Study the drawing (mm; zero at the part's minimum x, y, z) and answer. Coordinates: 2 decimals unless noted, no trailing zeros. Order: outer loops, then holes, each group sorted by start corner. A loop starts at its lowest first (then second) coordinate and runs counter-clockwise, first axis right, second up.
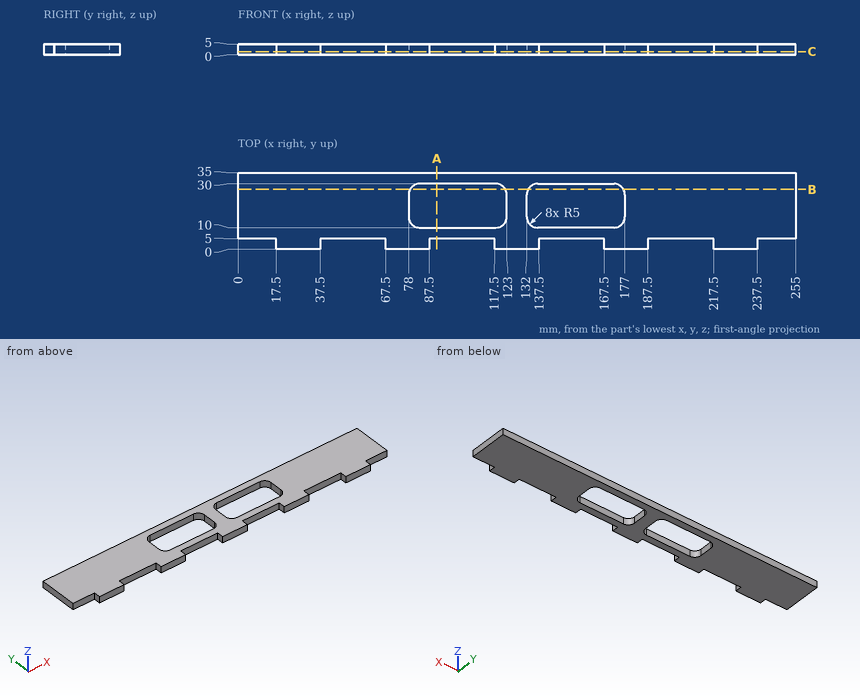
(1) Find the intervals of material crossed by probe 1 along X at (y, z) = (23.5, 2.3); probe 2 along X at (y, z) = (3.5, 4.1); probe 3 along Y at (x, z) = (97.5, 1.65), in increasing order.
(2) Given pin 1 Ø1.5 at (x, z) = (96, 1.5) entering from -Y; pin 2 Ø2.5 at (y, z) = (3.5, 3.5) entering from -X; pin 3 Ø2.5 at (y, z) = (3.5, 3) entering from +X, each flat-ended and moving along its own axis, determine where each tip first touches the part or whether it passes through.
(3) Find section B-B on y = 27.5. Determine the outline of the cut face in (x, z), then the cut area to 3 significant figures.
(4) Find section C-C on z = 1.5. Count the separate pieces of the cut face and the enclosed holes in it, then the cut area to 3 significant figures.
(5) Find section A-A on x = 91. Determine the outline of the cut face in (y, z).
Resolved:
1. probe 1: x = 0 to 78, 123 to 132, 177 to 255
1. probe 2: x = 17.5 to 37.5, 67.5 to 87.5, 117.5 to 137.5, 167.5 to 187.5, 217.5 to 237.5
1. probe 3: y = 5 to 10, 30 to 35
2. pin 1: stops at y = 5
2. pin 2: stops at x = 17.5
2. pin 3: stops at x = 237.5
3. outline: (0, 0) - (78.67, 0) - (78.67, 5) - (0, 5) - close; (122.33, 0) - (132.67, 0) - (132.67, 5) - (122.33, 5) - close; (176.33, 0) - (255, 0) - (255, 5) - (176.33, 5) - close
3. area: 838 mm2
4. separate pieces: 1
4. enclosed holes: 2
4. area: 6,390 mm2
5. outline: (5, 0) - (10, 0) - (10, 5) - (5, 5) - close; (30, 0) - (35, 0) - (35, 5) - (30, 5) - close
